from build123d import *

# Parameters (mm, degrees)
F0_R          = 63.5
F0_R_2        = 38.1
F1_DEPTH      = 127
F1_DEPTH_BACK = 127
F2_W          = 15.243814
F2_H          = 25.401894
F3_DEPTH      = 254.001


with BuildPart() as f1:
    # F0 (on Front) → F1 (new body, two sides)
    with BuildSketch(Plane.XZ) as f1_sk:
        Circle(F0_R)
        Circle(F0_R_2, mode=Mode.SUBTRACT)
    extrude(amount=F1_DEPTH)
    extrude(f1_sk.sketch, amount=-F1_DEPTH_BACK)

    # F2 (on face) → F3 (cut, through all)
    with BuildSketch(Plane.XZ.offset(127)):
        with Locations((0, 63.5)):
            Rectangle(F2_W, F2_H)
    extrude(amount=-F3_DEPTH, mode=Mode.SUBTRACT)


solid = f1.part
Could you check a few things on this model? Use its own coordinates, in mm. A direction names the side the tool comes from. Give positions to 0.01 mm unless a question says otherwise; leave off trailing zeros. Order: outer loops, then holes, each group sorted by start corner. A loop starts at its lowest first (then second) coordinate and runs counter-clockwise, first axis right, second up. Notation, with made-up numbers: (70.5, 16.5) - (122.5, 16.5) arc R33 cw to (122.5, 49.5) - close; hole circle Ø5 at (63.25, 18.5). An arc over 180 degrees is marked (long way). One line per item, written item: value. Start each with the question number.
1. If I drill on probe 1 along Z at (x, y) = (0, -12.5); probe 2 along Z at (x, y) = (-29, -116); probe 3 along X at (y, z) = (14, -22.5), over which ranges is the centre line in solid material (lowest first)?
2. Imagine slicing it at A-A on z = 0. List the corners of the cut face in (x, y) for me.
3. Thinking about a two-plate mould opening in X: for faces 3 (the face through (-2.685, -1.778, -63.443)), 4 (the face through (7.622, -2, 57)), 5 (the face through (27.3, 127, -27.5)), which applies, +X half, -X half, draft (parallel to the pull), parting line (faces both ways), or undercut?
4. For faces 1 (the face through (-7.622, -2, 57)), 2 (the face through (-30.235, 1.778, -23.183)), which set-ups out of +Z, -Z, +X, -X, +Y, -Y let a thin tool reach every point of the face, with its end or its side?
5. For P1, Ø10, axis at y = 30, z = 58.5, coming from the -X side; P2, Ø10, axis at y = -4.5, z = 60, coming from the +X side; P3, Ø12, axis at x = 4, y = 21, coming from the +Z side, each with a flat end and sliding along its axis, tell me the tip position at first contact or that it passes through.
6. Imagine slicing it at C-C on y = 49. List the corners of the cut face in (x, z) for me, plus the area to 3 significant figures.
7. Imagine slicing it at D-D on x = -55.5. List the corners of the cut face in (y, z) for me, plus the area to 3 significant figures.
8. Imagine slicing it at B-B on x = 0. List the corners of the cut face in (y, z) for me.
Values:
1. probe 1: -63.5 to -38.1, 38.1 to 50.8
1. probe 2: -56.49 to -24.71, 24.71 to 56.49
1. probe 3: -59.38 to -30.75, 30.75 to 59.38
2. outline: (-63.5, -127) - (-38.1, -127) - (-38.1, 127) - (-63.5, 127) - close; (38.1, -127) - (63.5, -127) - (63.5, 127) - (38.1, 127) - close
3. face 3: parting line
3. face 4: undercut
3. face 5: draft
4. face 1: +Z, +Y, -Y
4. face 2: +Y, -Y
5. P1: x = -34.21
5. P2: x = 31.74
5. P3: z = 63.04
6. outline: (-7.62, 50.8) - (-7.62, 63.04) arc R63.5 ccw (long way) to (7.62, 63.04) - (7.62, 50.8) - close; hole circle Ø76.2 at (0, 0)
6. area: 7,920 mm²
7. outline: (-127, -30.85) - (127, -30.85) - (127, 30.85) - (-127, 30.85) - close
7. area: 15,700 mm²
8. outline: (-127, -63.5) - (127, -63.5) - (127, -38.1) - (-127, -38.1) - close; (-127, 38.1) - (127, 38.1) - (127, 50.8) - (-127, 50.8) - close
